```python
from build123d import *

# Parameters (mm, degrees)
F0_R     = 33.899089
F0_R_2   = 10.977383
F1_DEPTH = 25.4


with BuildPart() as f1:
    # F0 (on Top) → F1 (new body)
    with BuildSketch(Plane.XY):
        with Locations((35.900313, 38.462833)):
            Circle(F0_R)
        with BuildLine():
            Line((29.684071, 23.595444), (31.375829, 23.595444))
            ThreePointArc((31.375829, 23.595444), (35.900313, 22.922234), (40.424798, 23.595444))
            Line((40.424798, 23.595444), (42.116555, 23.595444))
            Line((42.116555, 23.595444), (35.900313, 16.834289))
            Line((35.900313, 16.834289), (29.684071, 23.595444))
        make_face(mode=Mode.SUBTRACT)
        with BuildLine():
            Line((35.390319, 67.539793), (19.270614, 49.856011))
            Line((19.270614, 49.856011), (25.331222, 49.856011))
            ThreePointArc((25.331222, 49.856011), (20.379015, 39.237091), (24.249848, 28.178046))
            Line((24.249848, 28.178046), (18.442286, 28.178046))
            Line((18.442286, 28.178046), (35.390319, 9.385872))
            ThreePointArc((35.390319, 9.385872), (6.81888, 38.462833), (35.390319, 67.539793))
        make_face(mode=Mode.SUBTRACT)
        with Locations((35.900313, 38.462833)):
            Circle(F0_R_2, mode=Mode.SUBTRACT)
        with BuildLine():
            ThreePointArc((36.128241, 67.543372), (64.981746, 38.462833), (36.128241, 9.382293))
            Line((36.128241, 9.382293), (53.560682, 28.047737))
            Line((53.560682, 28.047737), (47.434436, 28.047737))
            ThreePointArc((47.434436, 28.047737), (51.434076, 38.923711), (46.796669, 49.543429))
            Line((46.796669, 49.543429), (53.530753, 49.543429))
            Line((53.530753, 49.543429), (36.128241, 67.543372))
        make_face(mode=Mode.SUBTRACT)
        with BuildLine():
            ThreePointArc((40.424798, 53.330221), (35.900313, 54.003431), (31.375829, 53.330221))
            Line((31.375829, 53.330221), (29.684071, 53.330221))
            Line((29.684071, 53.330221), (35.900313, 60.091376))
            Line((35.900313, 60.091376), (42.116555, 53.330221))
            Line((42.116555, 53.330221), (40.424798, 53.330221))
        make_face(mode=Mode.SUBTRACT)
    extrude(amount=F1_DEPTH)


solid = f1.part
```
Work out the finished part from the listing and answer in its coordinate system (mm). Round coordinates to 2 decimals unless told otherwise and drop trailing zeros. Loops run counter-clockwise (first coordinate to the right, second up) from the corner with the lowest first, then second, coordinate; pieces in that order, holes last. Notation, with made-up numbers: M -33.5,61.25 L 21.5,61.25 A24 cw 21.5,83.25 Z; hole C 74.5,31.5 d8. An arc over 180 degrees is marked long. One line per question, with ' | ' between items.
Q1. Find section B-B, the plane y = 14.5. Give the vertices of the cut face in (x, z), then the cut area to 3 significant figures.
Conclusion:
outline: M 11.92,0 L 19.42,0 L 19.42,25.4 L 11.92,25.4 Z; M 30.78,0 L 40.91,0 L 40.91,25.4 L 30.78,25.4 Z; M 52.38,0 L 59.88,0 L 59.88,25.4 L 52.38,25.4 Z | area: 638 mm2
Q2. The mould has two halves that part along Y. Classify faces 1 (the cylindrical face through (54.12, 67.05, 12.52)), 2 (the flat face through (26, 44, 0)), 3 (the flat face through (39.05, 20.26, 12.52)): +Y half, -Y half, draft (parallel to the pull), parting line (faces both ways), or undercut.
Conclusion:
face 1: parting line | face 2: draft | face 3: undercut
Q3. Find section C-C, the plane x = 46. Give the vertices of the cut face in (y, z), then the cut area to 3 significant figures.
Conclusion:
outline: M 6.1,0 L 11.19,0 L 11.19,25.4 L 6.1,25.4 Z; M 19.95,0 L 34.16,0 L 34.16,25.4 L 19.95,25.4 Z; M 42.76,0 L 57.33,0 L 57.33,25.4 L 42.76,25.4 Z; M 65.73,0 L 70.82,0 L 70.82,25.4 L 65.73,25.4 Z | area: 989 mm2
Q4. Find section A-A, the plane x = 14. Give the vertices of the cut face in (y, z).
Conclusion:
outline: M 12.59,0 L 19.33,0 L 19.33,25.4 L 12.59,25.4 Z; M 57.6,0 L 64.34,0 L 64.34,25.4 L 57.6,25.4 Z
Q5. Each of these flat-tipped pins is pushed along its axis until it touches: pin 1 Ø7.5 at (x, z) = (50.5, 13.5) entering from -Y; pin 2 Ø1.5 at (x, z) = (30, 5) entering from +Y; pin 3 Ø6.5 at (x, z) = (49.5, 9.5) entering from +Y; pin 4 Ø12 at (x, y) = (20.5, 12.5) entering from -Z. Where does it stop, or does it pass through?
Conclusion:
pin 1: stops at y = 6.35 | pin 2: stops at y = 71.97 | pin 3: stops at y = 70.74 | pin 4: stops at z = 0
Q6. Find section D-D, the plane z = 4. Give the vertices of the cut face in (x, y).
Conclusion:
outline: C 35.9,38.46 d67.8; hole M 18.44,28.18 L 24.25,28.18 A15.54 cw 25.33,49.86 L 19.27,49.86 L 35.39,67.54 A29.08 ccw 35.39,9.39 Z; hole C 35.9,38.46 d21.95; hole M 29.68,23.6 L 35.9,16.83 L 42.12,23.6 L 40.42,23.6 A15.54 cw 31.38,23.6 Z; hole M 29.68,53.33 L 31.38,53.33 A15.54 cw 40.42,53.33 L 42.12,53.33 L 35.9,60.09 Z; hole M 36.13,9.38 A29.08 ccw 36.13,67.54 L 53.53,49.54 L 46.8,49.54 A15.54 cw 47.43,28.05 L 53.56,28.05 Z
Q7. Consider line 1 along Y through (x, z) = (35, 23.5); line 2 along X through (y, z) = (48.5, 21.25); line 3 along X through (y, z) = (56, 4.25). Determine where each line is inside the solid, lowest interval first. Write a range as from..to.
Conclusion:
line 1: y = 4.58..9.4, 9.82..17.81, 22.95..27.52, 49.4..53.98, 59.11..67.11, 67.53..72.35 | line 2: x = 3.52..8.61, 24.04..31.46, 40.35..47.76, 63.19..68.28 | line 3: x = 6.89..12.7, 24.87..32.14, 39.66..47.29, 59.1..64.91
